The drawing under review shows one solid part. Ordinate dimensions are in mm from its lowest x, y, z. Give positions to 0.01 mm unless a question says otherwise; leave off trailing zeros. Order: outer loops, then holes, each group sorted by start corner. A loop starts at its lowest first (then second) coordinate and runs counter-clockwise, first axis right, second up. Notation, with made-up numbers: (47.5, -25.75) - (96.5, -25.75) arc R26 cw to (96.5, 10.25) - close; hole circle Ø7 at (40.5, 48.25). An arc over 180 degrees is marked (long way). Use CSV: the item, a comma, the result in double quotes.
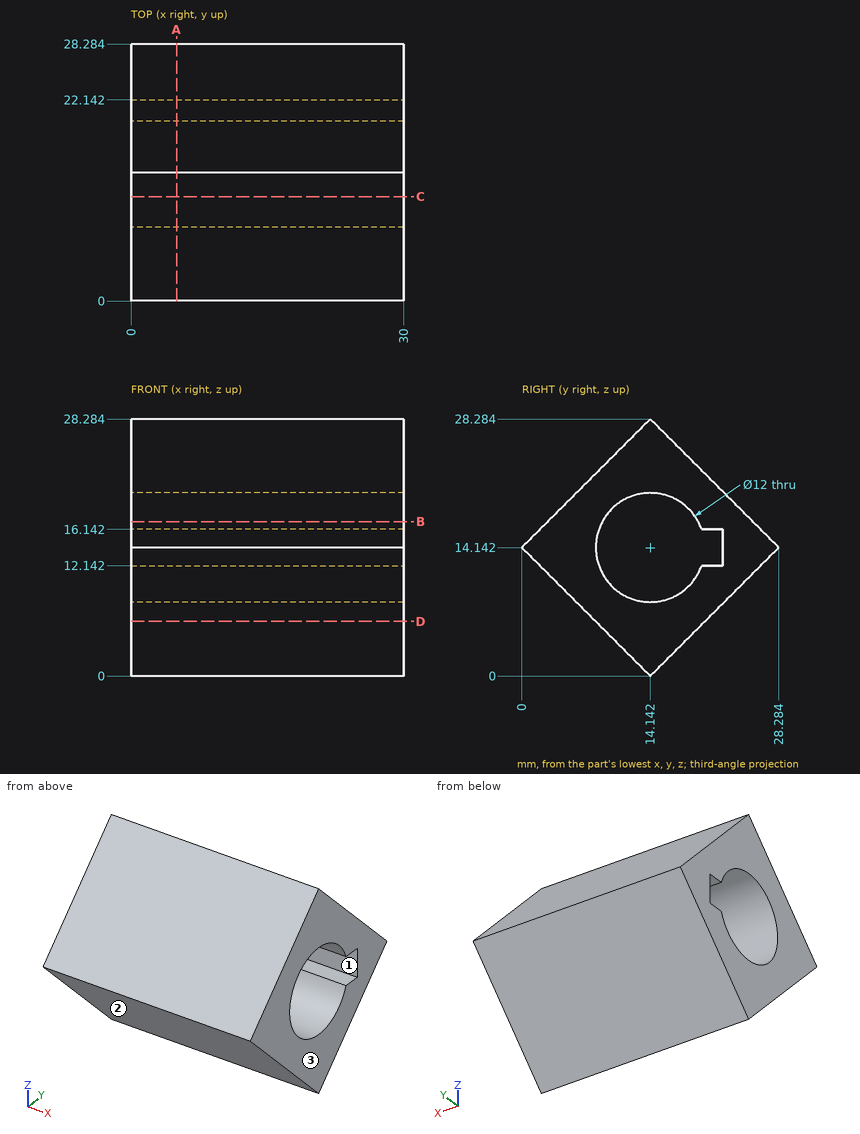
Item 1: Take a section at B-B, the plane z = 17. Give the boundary of the cut face in (x, y).
Results list:
outline,"(0, 2.86) - (30, 2.86) - (30, 8.87) - (0, 8.87) - close; (0, 19.42) - (30, 19.42) - (30, 25.43) - (0, 25.43) - close"
Item 2: Wall thickness on L1, parallel to Z at x = 9, y = 10; L2, parallel to Y at x = 25.5, z = 6; L3, parallel to Z at x = 10.5, y = 19 (1 decimal): over which ranges is each line inside the solid? List them lowest first.
Results list:
L1,"z = 4.14 to 9.8, 18.48 to 24.14"
L2,"y = 8.14 to 20.14"
L3,"z = 4.9 to 10.6, 17.7 to 23.4"
Item 3: Take a section at C-C, the plane y = 11.5. Give the boundary of the cut face in (x, z) (1 decimal).
Results list:
outline,"(0, 2.6) - (30, 2.6) - (30, 8.8) - (0, 8.8) - close; (0, 19.5) - (30, 19.5) - (30, 25.6) - (0, 25.6) - close"
Item 4: Take a section at D-D, the plane z = 6. Give the boundary of the cut face in (x, y).
Results list:
outline,"(0, 8.14) - (30, 8.14) - (30, 20.14) - (0, 20.14) - close"
Item 5: Take a section at A-A, the plane x = 5. Give the boundary of the cut face in (y, z).
Results list:
outline,"(0, 14.14) - (14.14, 0) - (28.28, 14.14) - (14.14, 28.28) - close; hole (19.8, 12.14) - (22.14, 12.14) - (22.14, 16.14) - (19.8, 16.14) arc R6 ccw (long way) to start"
Item 6: Clearance check with flat-ended pins moving along their axes: pin 1 (3 mm diameter, centred on x = 18.5, y = 23, fed in from -Z); pin 2 (1 mm diameter, centred on x = 18.5, z = 12, fed in from -Y); pin 3 (4.5 mm diameter, centred on x = 8, z = 13.5, fed in from -Y). State where each tip first meets the part, or that it passes through.
Results list:
pin 1,"stops at z = 7.36"
pin 2,"stops at y = 1.64"
pin 3,"stops at y = 0"
Item 7: Mouldability with a two-part tool opening along Y and no side actions: class the marked faces 1, 2 and 3 as pulls with the +Y half, pulls with the -Y half, needs draft (parallel to the pull), parting line crosses it, or undercut.
Results list:
face 1,"undercut"
face 2,"pulls with the -Y half"
face 3,"needs draft"
